CAD build for the part. Positions are in the model's coordinates, mm. A direction names the side the tool comes from. Coordinates: 2 decimals unless noted, no trailing zeros. Order: outer loops, then holes, each group sorted by start corner. A loop starts at its lowest first (then second) coordinate and runs counter-clockwise, first axis right, second up. Notation, with made-up numbers: M 0,-12 L 43,-12 A27 ccw 43,4 Z; hole C 35,-9.5 d10. An arc over 180 degrees is marked long. One line per item, written item: value.
from build123d import *

# Parameters (mm, degrees)
SKETCH1_W                       = 70.22
SKETCH1_H                       = 25.9
BOSS_EXTRUDE1_DEPTH             = 47.34
SKETCH6_W                       = 29.36
SKETCH6_H                       = 15.02
CUT_EXTRUDE1_DEPTH              = 65.378549999
SKETCH8_W                       = 57.62
SKETCH8_H                       = 41.04
CUT_EXTRUDE2_DEPTH              = 16.75
CUT_EXTRUDE3_DEPTH              = 86.671620155
CUT_EXTRUDE4_DEPTH              = 56.540041412
CUT_EXTRUDE4_DEPTH_BACK         = 56.540041412
FILLET9_R                       = 1
CBORE_FOR_M3_SBHCS1_D           = 3.4
CBORE_FOR_M3_SBHCS1_CBORE_D     = 6.7
CBORE_FOR_M3_SBHCS1_CBORE_DEPTH = 1.65
CBORE_FOR_M5_SBHCS1_D           = 5.5
CBORE_FOR_M5_SBHCS1_CBORE_D     = 10.5
CBORE_FOR_M5_SBHCS1_CBORE_DEPTH = 2.75


with BuildPart() as part:
    # Sketch1 → Boss-Extrude1 (new body)
    with BuildSketch(Plane.XY):
        Rectangle(SKETCH1_W, SKETCH1_H)
    extrude(amount=-BOSS_EXTRUDE1_DEPTH)

    # Sketch6 → Cut-Extrude1 (cut, through all)
    with BuildSketch(Plane(origin=(0, 12.95, 0), x_dir=(1, 0, 0), z_dir=(0, 1, 0))):
        with Locations((-20.43, 7.51)):
            Rectangle(SKETCH6_W, SKETCH6_H)
    cut_extrude1 = extrude(amount=-CUT_EXTRUDE1_DEPTH, mode=Mode.SUBTRACT)

    # Mirror1: Cut-Extrude1 across plane
    add(cut_extrude1.mirror(Plane(origin=(0, 0, 0), x_dir=(0, 0, 1), z_dir=(1, 0, 0))), mode=Mode.SUBTRACT)

    # Sketch8 → Cut-Extrude2 (cut)
    with BuildSketch(Plane(origin=(0, 12.95, 0), x_dir=(1, 0, 0), z_dir=(0, 1, 0))):
        with Locations((0, 20.52)):
            Rectangle(SKETCH8_W, SKETCH8_H)
    extrude(amount=-CUT_EXTRUDE2_DEPTH, mode=Mode.SUBTRACT)

    # Sketch12 → Cut-Extrude3 (cut, through all)
    with BuildSketch(Plane(origin=(35.11, 0, 0), x_dir=(0, 0, -1), z_dir=(1, 0, 0))):
        Polygon((15.02, -3.8), (41.04, 12.95), (15.02, 12.95), align=None)
    extrude(amount=-CUT_EXTRUDE3_DEPTH, mode=Mode.SUBTRACT)

    # Sketch16 → Cut-Extrude4 (cut, two sides: drawn at the far end of the back side and taken through both)
    with BuildSketch(Plane.XY.offset(-41.04).offset(-CUT_EXTRUDE4_DEPTH_BACK)):
        with BuildLine():
            Line((-7.395445113, 122.499442273), (-7.395445113, 12.95))
            ThreePointArc((-7.395445113, 12.95), (0, 5.554554887), (7.395445113, 12.95))
            Line((7.395445113, 12.95), (7.395445113, 122.499442273))
            Line((7.395445113, 122.499442273), (7.395445113, 341.598326819))
            Line((7.395445113, 341.598326819), (-7.395445113, 341.598326819))
            Line((-7.395445113, 341.598326819), (-7.395445113, 122.499442273))
        make_face()
    extrude(amount=CUT_EXTRUDE4_DEPTH + CUT_EXTRUDE4_DEPTH_BACK, mode=Mode.SUBTRACT)

    # Fillet9
    fillet9_edges = [part.edges().sort_by_distance(p)[0] for p in [
        (-35.11, 0, -47.34),
        (7.395445113, 12.95, -44.19),
        (-7.395445113, 12.95, -44.19),
        (-35.11, -8.375, -15.02),
        (35.11, -8.375, -15.02),
        (35.11, 0, -47.34),
        (-35.11, 12.95, -44.19),
        (35.11, 12.95, -44.19),
        (-35.11, 4.575, -28.03),
        (35.11, 4.575, -28.03),
    ]]
    fillet(fillet9_edges, radius=FILLET9_R)

    # CBORE for M3 SBHCS1 (through all)
    with Locations(Plane(origin=(0, 0, -47.34), x_dir=(-1, 0, 0), z_dir=(0, 0, -1))):
        with Locations((-15.61, 1.45), (15.61, 1.45)):
            CounterBoreHole(CBORE_FOR_M3_SBHCS1_D / 2, CBORE_FOR_M3_SBHCS1_CBORE_D / 2, CBORE_FOR_M3_SBHCS1_CBORE_DEPTH)

    # CBORE for M5 SBHCS1 (through all)
    with Locations(Plane.XZ.offset(12.95)):
        with Locations((-25.11, -28.02), (25.11, -28.02)):
            CounterBoreHole(CBORE_FOR_M5_SBHCS1_D / 2, CBORE_FOR_M5_SBHCS1_CBORE_D / 2, CBORE_FOR_M5_SBHCS1_CBORE_DEPTH)


solid = part.part
Q1. Slice it at A-A (x = 15.61). List the corners of the cut face in (y, z).
Recorded:
outline: M -12.95,-47.34 L -1.9,-47.34 L -1.9,-45.69 L -0.25,-45.69 L -0.25,-41.04 L -3.8,-41.04 L -3.8,-15.02 L -12.95,-15.02 Z; M 3.15,-45.69 L 4.8,-45.69 L 4.8,-47.34 L 12.95,-47.34 L 12.95,-41.04 L 3.15,-41.04 Z
Q2. Slice it at B-B (y = -6.75). List the corners of the cut face in (x, z), plus the area to 3 significant figures.
Recorded:
outline: M -35.11,-46.34 A1 ccw -34.11,-47.34 L 34.11,-47.34 A1 ccw 35.11,-46.34 L 35.11,-16.02 A1 ccw 34.11,-15.02 L 5.75,-15.02 L 5.75,0 L -5.75,0 L -5.75,-15.02 L -34.11,-15.02 A1 ccw -35.11,-16.02 Z; hole C -25.11,-28.02 d5.5; hole C 25.11,-28.02 d5.5
area: 2,390 mm^2
Q3. Slice it at C-C (x = -25.11). List the corners of the cut face in (y, z).
Recorded:
outline: M -12.95,-47.34 L 12.95,-47.34 L 12.95,-41.04 L -3.8,-41.04 L -3.8,-30.77 L -10.2,-30.77 L -10.2,-33.27 L -12.95,-33.27 Z; M -12.95,-22.77 L -10.2,-22.77 L -10.2,-25.27 L -3.8,-25.27 L -3.8,-15.02 L -12.95,-15.02 Z
Q4. Pin check, flat tips, straight feed: pin 1 Ø7.5 at (x, y) = (-16, -10.5) entering from +Z; pin 2 Ø5 at (x, z) = (25.11, -28.02) entering from +Y; pin 3 Ø8.5 at (y, z) = (8, -28) entering from +X; pin 4 Ø10 at (y, z) = (-8.5, -5) entering from -X. Stop position of each tip, or through.
Recorded:
pin 1: stops at z = -15.02
pin 2: passes through
pin 3: stops at x = 35.11
pin 4: stops at x = -5.75
Q5. Drill centre lines: line 1 along Z through (x, y) = (-25.11, -11.1); line 2 along Y through (x, z) = (-15.61, -43); line 3 along Z through (x, y) = (-25.11, -8.5). Where is each one in solid material? Low to high.
Recorded:
line 1: z = -47.34 to -33.27, -22.77 to -15.02
line 2: y = -12.95 to -0.25, 3.15 to 12.95
line 3: z = -47.34 to -30.77, -25.27 to -15.02
Q6. Which spindle directions (+Z, -Z, +X, -X, +Y, -Y) get a long thin tool onto all of the face, cutting with end or side? Do faces 4 (the face through (-5.75, -8, -7)), 5 (the face through (-13.141, 3.714, -46.527)), 6 (the face through (-28.81, 1, -34)), 7 (the face through (30.118, -11.594, -26.443)). Say none if no direction does.
Recorded:
face 4: +Z, -X, +Y, -Y
face 5: -Z
face 6: +Z, +Y
face 7: -Y
Q7. Mould opens along Z. For faces 1 (the face through (21, 12.95, -44)), 2 (the face through (-22.9, -10.2, -30.3)), 3 (the face through (0, 5, -41.04)) say: released by +Z, released by -Z, zero draft, split by the parting line, or undercut.
Recorded:
face 1: zero draft
face 2: undercut
face 3: released by +Z
Q8. Slice it at D-D (z = -28.02). Give the number of separate pieces and of enclosed holes in the cut face, plus the area to 3 significant figures.
Recorded:
separate pieces: 3
enclosed holes: 0
area: 619 mm^2
